```python
from build123d import *

# Parameters (mm, degrees)
F0_W     = 279.4
F0_H     = 101.6
F0_R     = 3.175
F1_DEPTH = 101.6
F2_W     = 6.35
F2_H     = 101.6
F3_DEPTH = 12.7
F4_W     = 292.1
F4_H     = 114.3
F4_W_2   = 50.6314568898
F4_H_2   = 101.5523529232
F4_W_3   = 50.8
F4_H_3   = 101.6
F5_DEPTH = 25.4


with BuildPart() as f1:
    # F0 (on Top) → F1 (new body)
    with BuildSketch(Plane.XY):
        with Locations((9.3390280625, 1.3603759766)):
            Rectangle(F0_W, F0_H)
        with Locations((-104.9609719375, -30.3896240234)):
            Circle(F0_R, mode=Mode.SUBTRACT)
        with Locations((-47.8109719375, -30.3896240234)):
            Circle(F0_R, mode=Mode.SUBTRACT)
        with Locations((9.3390280625, -30.3896240234)):
            Circle(F0_R, mode=Mode.SUBTRACT)
        with Locations((66.4890280625, -30.3896240234)):
            Circle(F0_R, mode=Mode.SUBTRACT)
        with Locations((-104.9609719375, 1.3603759766)):
            Circle(F0_R, mode=Mode.SUBTRACT)
        with Locations((-47.8109719375, 1.3603759766)):
            Circle(F0_R, mode=Mode.SUBTRACT)
        with Locations((-104.9609719375, 33.1103759766)):
            Circle(F0_R, mode=Mode.SUBTRACT)
        with Locations((-47.8109719375, 33.1103759766)):
            Circle(F0_R, mode=Mode.SUBTRACT)
        with Locations((9.3390280625, 1.3603759766)):
            Circle(F0_R, mode=Mode.SUBTRACT)
        with Locations((66.4890280625, 1.3603759766)):
            Circle(F0_R, mode=Mode.SUBTRACT)
        with Locations((9.3390280625, 33.1103759766)):
            Circle(F0_R, mode=Mode.SUBTRACT)
        with Locations((66.4890280625, 33.1103759766)):
            Circle(F0_R, mode=Mode.SUBTRACT)
    extrude(amount=F1_DEPTH)

    # F2 (on face) → F3 (cut)
    with BuildSketch(Plane.XY.offset(101.6)):
        with Locations((-76.3859719375, 1.3603759766)):
            Rectangle(F2_W, F2_H)
        with Locations((-19.2359719375, 1.3603759766)):
            Rectangle(F2_W, F2_H)
        with Locations((37.9140280625, 1.3603759766)):
            Rectangle(F2_W, F2_H)
        with Locations((95.0640280625, 1.3603759766)):
            Rectangle(F2_W, F2_H)
    extrude(amount=-F3_DEPTH, mode=Mode.SUBTRACT)

    # F4 (on face) → F5 (join)
    with BuildSketch(Plane.XY.offset(88.9)):
        with Locations((9.3390280625, 1.3603759766)):
            Rectangle(F4_W, F4_H)
        with Locations((-104.8767003824, 1.3365524381)):
            Rectangle(F4_W_2, F4_H_2, mode=Mode.SUBTRACT)
        with Locations((-47.8109719375, 1.3603759766)):
            Rectangle(F4_W_3, F4_H_3, mode=Mode.SUBTRACT)
        with Locations((9.3390280625, 1.3603759766)):
            Rectangle(F4_W_3, F4_H_3, mode=Mode.SUBTRACT)
        with Locations((66.4890280625, 1.3603759766)):
            Rectangle(F4_W_3, F4_H_3, mode=Mode.SUBTRACT)
        with Locations((123.6390280625, 1.3603759766)):
            Rectangle(F4_W_3, F4_H_3, mode=Mode.SUBTRACT)
    extrude(amount=F5_DEPTH)


solid = f1.part
```
CAD build for the part. Positions are in the model's coordinates, mm. A direction names the side the tool comes from. Coordinates: 2 decimals unless noted, no trailing zeros. Write each loop counter-clockwise with the first axis right and the second up, starting at its lowest first coordinate (ties: lowest second). Pieces come first, ordered by that corner, then holes.
(1) Cut at C-C, the plane x = -56. List the corners of the cut face in (y, z), and give its area (3 significant figures).
(2) Cut at A-A, the plane z = 10.5. Count the separate pieces of the cut face and the enclosed holes in it, and give its area (3 significant figures).
(3) 3-axis set-ups, long thin cutter, end or side, ignore diameter. For faces 5 (the face through (7, 13, 0)), 6 (the face through (9, -49.44, 108)), 7 (the face through (7, 52.16, 44)): which of +Z, -Z, +X, -X, +Y, -Y reach the whole face in a straight line?
(4) Drill centre lines: probe 1 along X at (y, z) = (-45, 109); probe 2 along X at (y, z) = (1, 27); probe 3 along X at (y, z) = (36, 92). Where is each one in solid material? Low to high.
(5) Flat gauge pins, fed straight in: pin 1 (4 mm diameter, centred on x = 5.5, z = 52.5, fed in from +Y); pin 2 (2 mm diameter, centred on x = -75, z = 73, fed in from -Y); pin 3 (10 mm diameter, centred on x = -34, y = -15.5, fed in from +Z); pin 4 (8.5 mm diameter, centred on x = -47.81, y = 1.36, fed in from -Z). Where does each tip first touch, or does it go through?
(6) Cut at B-B, the plane y = 48.5. List the corners of the cut face in (x, z), and give its area (3 significant figures).
(7) Two-plate mould, pull along X, no slides. Class faces 1 (the face through (149.039, 1, 44)), 2 (the face through (-136.711, 1, 101)), 3 (the face through (8.7, 52.4, 114.3)), 4 (the face through (123, 52.16, 108)): +X half, -X half, draft (parallel to the pull), parting line (faces both ways), or undercut.
Geometry says:
1. outline: (-55.79, 88.9) - (-49.44, 88.9) - (-49.44, 0) - (52.16, 0) - (52.16, 88.9) - (58.51, 88.9) - (58.51, 114.3) - (52.16, 114.3) - (52.16, 101.6) - (-49.44, 101.6) - (-49.44, 114.3) - (-55.79, 114.3) - close
1. area: 10,600 mm2
2. separate pieces: 1
2. enclosed holes: 12
2. area: 28,000 mm2
3. face 5: -Z, +X, -X, +Y, -Y
3. face 6: +Z
3. face 7: -Z, +X, -X, +Y
4. probe 1: x = -136.71 to -130.19, -79.56 to -73.21, -22.41 to -16.06, 34.74 to 41.09, 91.89 to 98.24, 149.04 to 155.39
4. probe 2: x = -130.36 to -108.12, -101.81 to -50.97, -44.66 to 6.18, 12.49 to 63.33, 69.64 to 149.04
4. probe 3: x = -136.71 to -106.28, -103.65 to -49.13, -46.5 to 8.02, 10.65 to 65.17, 67.8 to 155.39
5. pin 1: stops at y = 52.16
5. pin 2: stops at y = -49.44
5. pin 3: stops at z = 101.6
5. pin 4: stops at z = 0
6. outline: (-136.71, 88.9) - (-130.36, 88.9) - (-130.36, 0) - (149.04, 0) - (149.04, 88.9) - (155.39, 88.9) - (155.39, 114.3) - (149.04, 114.3) - (149.04, 101.6) - (98.24, 101.6) - (98.24, 114.3) - (91.89, 114.3) - (91.89, 101.6) - (41.09, 101.6) - (41.09, 114.3) - (34.74, 114.3) - (34.74, 101.6) - (-16.06, 101.6) - (-16.06, 114.3) - (-22.41, 114.3) - (-22.41, 101.6) - (-73.21, 101.6) - (-73.21, 114.3) - (-79.56, 114.3) - (-79.56, 101.6) - (-130.19, 101.6) - (-130.19, 114.3) - (-136.71, 114.3) - close
6. area: 29,000 mm2
7. face 1: +X half
7. face 2: -X half
7. face 3: draft
7. face 4: undercut
